Check sheet for the modelled part. Datum: model origin and axes. Units: mm. A direction names the side the tool comes from. Coordinates: 2 decimals unless noted, no trailing zeros. Write each loop counter-clockwise with the first axis right and the second up, starting at its lowest first coordinate (ties: lowest second). Pieces come first, ordered by that corner, then holes. Notation, with made-up numbers: (2.25, -14) -> (9.25, -14) arc R14 cw to (9.25, 0) -> close; hole circle Ø10 at (67.25, -14). An arc over 180 degrees is marked (long way). One line per item, written item: value. Start each with the question number.
1) Draft check along X on faces 4 (the flat face through (400, -534, -116)), 5 (the flat face through (385, -412, 180)), 6 (the cylindrical face through (305.63, -266.234, 18.876)). Enter one of: +X half, -X half, draft (parallel to the pull), parting line (faces both ways), or undercut.
2) Gauge pin test, flat ends, axial feed: P1, Ø8, axis at x = -50.5, y = -316.5, coming from the +Z side; P2, Ø24, axis at y = -540, z = -130, coming from the -X side; P3, Ø4, axis at x = 194.5, y = -511.5, coming from the -Z side; P4, Ø5, axis at x = 311.5, z = -117.5, coming from the -Y side. Record the tip position at first contact, or that the pin passes through.
3) Scan lines: line 1 along Y through (x, z) = (379, 130); line 2 along Z through (x, y) = (402, -540); line 3 along X through (y, z) = (-35.5, 130). Record each from-to range of solid material in increasing order. Write a range as [from, to].
4) Sectioned sample at B-B on y = -280. Give the number of separate pieces and of enclosed holes in the cut face, plus the area to 3 significant figures.
5) Set-up check for faces 1 (the flat face through (400, -286, -144)), 2 (the flat face through (157, -50, -3)), 3 (the flat face through (385, -230, 2)): record each of +Z, -Z, +X, -X, +Y, -Y from which the full face is reachable in a straight line by a thin tool's end or side.
6) Sectioned sample at A-A on x = 269.5. Enter the section's corners in (y, z), plus the area to 3 significant figures.
```python
from build123d import *

# Parameters (mm, degrees)
SKETCH1_W           = 360
SKETCH1_H           = 360
SKETCH1_R           = 105
SKETCH1_R_2         = 15
BOSS_EXTRUDE1_DEPTH = 50
SKETCH2_R           = 30
CUT_EXTRUDE1_DEPTH  = 10
CHAMFER1_SIZE       = 10
SKETCH3_R           = 145
BOSS_EXTRUDE2_DEPTH = 100
SKETCH5_R           = 105
CUT_EXTRUDE2_DEPTH  = 100
FILLET1_R           = 10
FILLET2_R           = 20
SWEEP4_OUTLINE_R    = 145
SWEEP4_OUTLINE_R_2  = 105
SWEEP4_ANGLE        = 45


# Read off the part's stored shape, not the designer's step: Sweep4
with BuildPart() as part:
    # Sketch1 → Boss-Extrude1 (new body)
    with BuildSketch(Plane(origin=(0, 0, 0), x_dir=(1, 0, 0), z_dir=(0, 1, 0))):
        Rectangle(SKETCH1_W, SKETCH1_H)
        with Locations(Location((0, 0, 0), (0, 0, 270))):
            Circle(SKETCH1_R, mode=Mode.SUBTRACT)
        with Locations(Location((-130, -130, 0), (0, 0, 270))):
            Circle(SKETCH1_R_2, mode=Mode.SUBTRACT)
        with Locations(Location((130, -130, 0), (0, 0, 90))):
            Circle(SKETCH1_R_2, mode=Mode.SUBTRACT)
        with Locations(Location((130, 130, 0), (0, 0, 270))):
            Circle(SKETCH1_R_2, mode=Mode.SUBTRACT)
        with Locations(Location((-130, 130, 0), (0, 0, 90))):
            Circle(SKETCH1_R_2, mode=Mode.SUBTRACT)
    extrude(amount=-BOSS_EXTRUDE1_DEPTH)

    # Sketch2 → Cut-Extrude1 (cut)
    with BuildSketch(Plane(origin=(0, 0, 0), x_dir=(1, 0, 0), z_dir=(0, 1, 0))):
        with Locations(Location((-130, -130, 0), (0, 0, 270))):
            Circle(SKETCH2_R)
        with Locations(Location((130, -130, 0), (0, 0, 90))):
            Circle(SKETCH2_R)
        with Locations(Location((130, 130, 0), (0, 0, 270))):
            Circle(SKETCH2_R)
        with Locations(Location((-130, 130, 0), (0, 0, 90))):
            Circle(SKETCH2_R)
    extrude(amount=-CUT_EXTRUDE1_DEPTH, mode=Mode.SUBTRACT)

    # Chamfer1
    chamfer1_edges = [part.edges().sort_by_distance(p)[0] for p in [
        (0, 0, -105),
    ]]
    chamfer(chamfer1_edges, length=CHAMFER1_SIZE)

    # Sketch3 → Boss-Extrude2 (add)
    with BuildSketch(Plane.XZ.offset(50)):
        with Locations(Location((0, 0, 0), (0, 0, 270))):
            Circle(SKETCH3_R)
    extrude(amount=BOSS_EXTRUDE2_DEPTH)

    # Sketch5 → Cut-Extrude2 (cut)
    with BuildSketch(Plane(origin=(0, -50, 0), x_dir=(1, 0, 0), z_dir=(0, 1, 0))):
        with Locations(Location((0, 0, 0), (0, 0, 270))):
            Circle(SKETCH5_R)
    extrude(amount=-CUT_EXTRUDE2_DEPTH, mode=Mode.SUBTRACT)

    # Fillet1
    fillet1_edges = [part.edges().sort_by_distance(p)[0] for p in [
        (0, -50, 145),
    ]]
    fillet(fillet1_edges, radius=FILLET1_R)

    # Fillet2
    fillet2_edges = [part.edges().sort_by_distance(p)[0] for p in [
        (180, -25, 180),
        (-180, -25, 180),
        (-180, -25, -180),
        (180, -25, -180),
    ]]
    fillet(fillet2_edges, radius=FILLET2_R)

    # Sweep4 outline → Sweep4 (revolve)
    with BuildSketch(Plane(origin=(260, -150, 0), x_dir=(-1, 0, 0), z_dir=(0, 1, 0))):
        with Locations((260, 0)):
            Circle(SWEEP4_OUTLINE_R)
        with Locations((260, 0)):
            Circle(SWEEP4_OUTLINE_R_2, mode=Mode.SUBTRACT)
    revolve(axis=Axis((260, -150, 0), (0, 0, 1)), revolution_arc=SWEEP4_ANGLE)

    # Mirror2: part across plane


with BuildPart() as part_1:
    add(part.part)
    add(part.part.mirror(Plane(origin=(76.152236891, -333.847763109, 0), x_dir=(0, 0, 1), z_dir=(0.7071067811865438, -0.7071067811865512, 0))))


solid = part_1.part
```
Answers:
1. face 4: +X half
1. face 5: draft
1. face 6: undercut
2. P1: stops at z = 114.99
2. P2: passes through
2. P3: stops at z = -99.59
2. P4: stops at y = -498.32
3. line 1: y = [-590, -555], [-525, -295], [-265, -230]
3. line 2: z = [-180, -160], [-100, 100], [160, 180]
3. line 3: x = [-180, -145], [-115, 115], [145, 180]
4. separate pieces: 3
4. enclosed holes: 1
4. area: 71,700 mm2
5. face 1: +X
5. face 2: none
5. face 3: +Z, -Z, +X, +Y
6. outline: circle Ø290 at (-410, 0); hole circle Ø210 at (-410, 0)
6. area: 31,400 mm2
